Part model, mm, in its own coordinate system. Face numbers are marked on the shaded views. Coordinates: 2 decimals unless noted, no trailing zeros. Write each loop counter-clockwise with the first axis right and the second up, starting at its lowest first coordinate (ties: lowest second). Pieces come first, ordered by that corner, then holes. Notation, with made-up numbers: M -1,-9 L 9,-9 A26 cw 9,6 Z; hole C -10.75,6.25 d11. An arc over 180 degrees is marked long. Use a Markdown table: item, result. Add a question column.
Q1. Slice it at B-B on x = 43.5. Write the cut outline in (y, z), then the cut area to 3 significant figures.
Q2. Mould opens along Y. For the marked faces 1, 2, 3 and 4 say: released by +Y, released by -Y, zero draft, split by the parting line, or undercut.
Q3. Slice it at A-A on y = 7.5. Write the cut outline in (x, z).
Q4. Slice it at D-D on z = 4. Write the cut outline in (x, y), then the cut area to 3 significant figures.
Q5. Slice it at C-C on z = 7. Write the cut outline in (x, y), then the cut area to 3 significant figures.
Q6. Wall check: L1, parallel to Y at x = 6.5, z = 4.5; L2, parallel to X at y = 1.5, z = 7.5; L3, parallel to X at y = 6, z = 4. Give the ranges that are in metal, low to high. Write a range as from..to.
Q7. Pin check, flat tip, straight feed: pin 1 Ø3.5 at (x, y) = (6.5, 7.5) entering from -Z. Stop position of the tip, or through.
from build123d import *

# Parameters (mm, degrees)
SKETCH1_W           = 50
SKETCH1_H           = 15
BOSS_EXTRUDE1_DEPTH = 14
SKETCH2_R           = 2.5
CUT_EXTRUDE1_DEPTH  = 16
SKETCH3_R           = 2.25
CUT_EXTRUDE2_DEPTH  = 15


with BuildPart() as part:
    # Sketch1 → Boss-Extrude1 (new body)
    with BuildSketch(Plane.XY):
        with Locations((25, 7.5)):
            Rectangle(SKETCH1_W, SKETCH1_H)
    extrude(amount=BOSS_EXTRUDE1_DEPTH)

    # Sketch2 → Cut-Extrude1 (cut, through all)
    with BuildSketch(Plane(origin=(0, 15, 0), x_dir=(1, 0, 0), z_dir=(0, 1, 0))):
        with Locations((32, -7.541991602)):
            Circle(SKETCH2_R)
    extrude(amount=-CUT_EXTRUDE1_DEPTH, mode=Mode.SUBTRACT)

    # Sketch3 → Cut-Extrude2 (cut, through all)
    with BuildSketch(Plane.XY.offset(14)):
        with Locations((6.5, 7.5)):
            Circle(SKETCH3_R)
        with Locations((43.5, 7.5)):
            Circle(SKETCH3_R)
    extrude(amount=-CUT_EXTRUDE2_DEPTH, mode=Mode.SUBTRACT)


solid = part.part
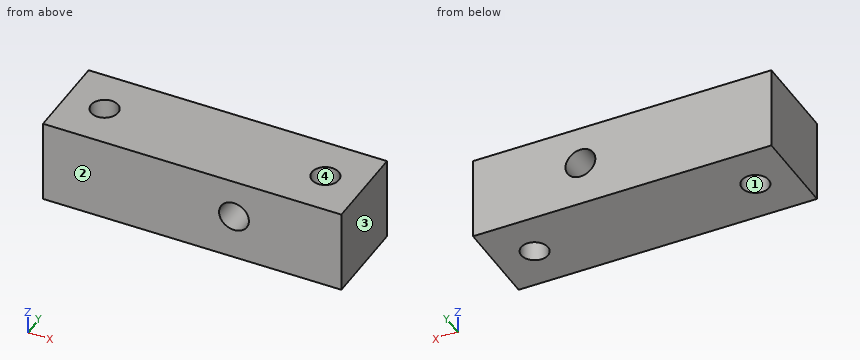
Recorded:
| question | item | result |
|---|---|---|
| 1 | outline | M 0,0 L 5.25,0 L 5.25,14 L 0,14 Z; M 9.75,0 L 15,0 L 15,14 L 9.75,14 Z |
| 1 | area | 147 mm² |
| 2 | face 1 | undercut |
| 2 | face 2 | released by -Y |
| 2 | face 3 | zero draft |
| 2 | face 4 | undercut |
| 3 | outline | M 0,0 L 4.25,0 L 4.25,14 L 0,14 Z; M 8.75,0 L 41.25,0 L 41.25,14 L 8.75,14 Z; M 45.75,0 L 50,0 L 50,14 L 45.75,14 Z; hole C 32,7.54 d5 |
| 4 | outline | M 0,0 L 50,0 L 50,15 L 0,15 Z; hole C 6.5,7.5 d4.5; hole C 43.5,7.5 d4.5 |
| 4 | area | 718 mm² |
| 5 | outline | M 0,0 L 29.56,0 L 29.56,15 L 0,15 Z; M 34.44,0 L 50,0 L 50,15 L 34.44,15 Z; hole C 6.5,7.5 d4.5; hole C 43.5,7.5 d4.5 |
| 5 | area | 645 mm² |
| 6 | L1 | 0..5.25, 9.75..15 |
| 6 | L2 | 0..29.5, 34.5..50 |
| 6 | L3 | 0..4.82, 8.18..41.82, 45.18..50 |
| 7 | pin 1 | through |
